from build123d import *
from build123d.topology import SkipClean

# Parameters (mm, degrees)
SKETCH1_R           = 15
SKETCH1_R_2         = 1.6
BOSS_EXTRUDE1_DEPTH = 7
BOSS_EXTRUDE2_DEPTH = 7.42
SKETCH3_R           = 9.5
BOSS_EXTRUDE3_DEPTH = 12.88
SKETCH5_R           = 1.6
CUT_EXTRUDE1_DEPTH  = 20
SKETCH6_R           = 2.75
CUT_EXTRUDE2_DEPTH  = 16
FILLET1_R           = 2
CHAMFER1_SIZE       = 0.4


with BuildPart() as part:
    # Sketch1 → Boss-Extrude1 (new body)
    with BuildSketch(Plane(origin=(0, 0, 0), x_dir=(1, 0, 0), z_dir=(0, 1, 0))):
        with Locations(Location((0, 0, 0), (0, 0, 270))):
            Circle(SKETCH1_R)
        with Locations(Location((0, 10, 0), (0, 0, 270))):
            Circle(SKETCH1_R_2, mode=Mode.SUBTRACT)
        with Locations(Location((0, -10, 0), (0, 0, 270))):
            Circle(SKETCH1_R_2, mode=Mode.SUBTRACT)
        with Locations(Location((10, 0, 0), (0, 0, 270))):
            Circle(SKETCH1_R_2, mode=Mode.SUBTRACT)
        with Locations(Location((-10, 0, 0), (0, 0, 270))):
            Circle(SKETCH1_R_2, mode=Mode.SUBTRACT)
    extrude(amount=BOSS_EXTRUDE1_DEPTH)

    # Sketch2 → Boss-Extrude2 (add)
    with BuildSketch(Plane(origin=(0, 7, 0), x_dir=(1, 0, 0), z_dir=(0, 1, 0))):
        Polygon((-6.505, 10.155), (6.505, 10.155), (10.155, 6.505), (10.155, -6.505), (6.505, -10.155), (-6.505, -10.155), (-10.155, -6.505), (-10.155, 6.505), align=None)
    extrude(amount=BOSS_EXTRUDE2_DEPTH)

    # Sketch3 → Boss-Extrude3 (add)
    with BuildSketch(Plane(origin=(0, 14.42, 0), x_dir=(1, 0, 0), z_dir=(0, 1, 0))):
        with Locations(Location((0, 0, 0), (0, 0, 90))):
            Circle(SKETCH3_R)
    extrude(amount=BOSS_EXTRUDE3_DEPTH)

    # Sketch4 → Cut-Revolve1 (revolve, cut)
    with BuildSketch(Plane.XY, mode=Mode.PRIVATE) as cut_revolve1_sk:
        Polygon((9, 25.05), (10, 25.05), (10, 26.05), (9.5, 26.05), (9, 25.761324865), align=None)
    revolve(cut_revolve1_sk.sketch.rotate(Axis((0, 27.3, 0), (0, -1, 0)), 270), axis=Axis((0, 27.3, 0), (0, -1, 0)), mode=Mode.SUBTRACT)

    # Sketch5 → Cut-Extrude1 (cut)
    with SkipClean():  # the faces are left unmerged after this step: merging them gives an invalid solid
        with BuildSketch(Plane.XZ):
            with Locations(Location((0, -10, 0), (0, 0, 185.559247246))):
                Circle(SKETCH5_R)
            with Locations(Location((10, 0, 0), (0, 0, 275.559247246))):
                Circle(SKETCH5_R)
            with Locations(Location((-10, 0, 0), (0, 0, 264.440752754))):
                Circle(SKETCH5_R)
            with Locations(Location((0, 10, 0), (0, 0, 202.624341254))):
                Circle(SKETCH5_R)
        extrude(amount=-CUT_EXTRUDE1_DEPTH, mode=Mode.SUBTRACT)

    # Sketch6 → Cut-Extrude2 (cut)
    with BuildSketch(Plane.XZ.offset(-20)):
        with Locations(Location((10, 0, 0), (0, 0, 90))):
            Circle(SKETCH6_R)
        with Locations(Location((0, 10, 0), (0, 0, 90))):
            Circle(SKETCH6_R)
        with Locations(Location((-10, 0, 0), (0, 0, 90))):
            Circle(SKETCH6_R)
        with Locations(Location((0, -10, 0), (0, 0, 90))):
            Circle(SKETCH6_R)
    extrude(amount=CUT_EXTRUDE2_DEPTH, mode=Mode.SUBTRACT)

    # Fillet1
    fillet1_edges = [part.edges().sort_by_distance(p)[0] for p in [
        (7.25, 20, 0),
        (0, 20, 7.25),
        (-7.25, 20, 0),
        (-1.609663202, 20, -7.770317427),
    ]]
    fillet(fillet1_edges, radius=FILLET1_R)

    # Chamfer1
    chamfer1_edges = [part.edges().sort_by_distance(p)[0] for p in [
        (0, 27.3, 9.5),
    ]]
    chamfer(chamfer1_edges, length=CHAMFER1_SIZE)


solid = part.part
Design review of the part built by this model. Coordinates are the model's own, in mm. A direction names the side the tool comes from. Round coordinates to 2 decimals unless told otherwise and drop trailing zeros. Order: outer loops, then holes, each group sorted by start corner. A loop starts at its lowest first (then second) coordinate and runs counter-clockwise, first axis right, second up.
1) For L1, parallel to Y at x = -5.75, z = -12; L2, parallel to X at y = 21.25, z = 0; L3, parallel to Y at x = 9.25, z = 5.5, list the stretches that pass through material, from the lowest coordinate up.
The answers:
L1: y = 0 to 7
L2: x = -9.5 to 9.5
L3: y = 0 to 14.42
2) Clearance check with flat-ended pins moving along their axes: pin 1 Ø8.5 at (x, z) = (7, 8) entering from +Y; pin 2 Ø3 at (x, y) = (4.5, 10) entering from -Z (3 decimals); pin 3 Ø8 at (x, y) = (2.5, 17) entering from +Z (3 decimals); pin 4 Ø3 at (y, z) = (9.5, -4) entering from -X (3 decimals). State where each tip first meets the part, or that it passes through.
The answers:
pin 1: stops at y = 27.3
pin 2: stops at z = -10.155
pin 3: stops at z = 10.155
pin 4: stops at x = -10.155
3) Consider section C-C (y = 16). State the section outline as (x, z) points, plus the area to 3 significant figures.
The answers:
outline: (-9.13, -2.61) arc R9.5 ccw to (-2.61, -9.13) arc R2.75 cw to (2.61, -9.13) arc R9.5 ccw to (9.13, -2.61) arc R2.75 cw to (9.13, 2.61) arc R9.5 ccw to (2.61, 9.13) arc R2.75 cw to (-2.61, 9.13) arc R9.5 ccw to (-9.13, 2.61) arc R2.75 cw to start
area: 250 mm2
4) Consider section D-D (y = 23.75). State the section outline as (x, z) points, plus the area to 3 significant figures.
The answers:
outline: circle Ø19 at (0, 0)
area: 284 mm2
5) Consider section A-A (z = 0). Count the separate pieces of the cut face and the enclosed holes in it, plus the area to 3 significant figures.
The answers:
separate pieces: 3
enclosed holes: 0
area: 479 mm2
6) Draft analysis for pull direction Y (two halves, no side actions). For faces 6 (the flat face through (10, 7, -7)), 7 (the flat face through (5, 11, -10.155)), 8 (the cylindrical face through (-0.83, 9.54, -7.38)), state which applies: released by +Y, released by -Y, zero draft, split by the parting line, or undercut.
The answers:
face 6: released by +Y
face 7: zero draft
face 8: undercut
7) Machinability: for faces 1 (the flat face through (-7, 14.42, 7)), 2 (the flat face through (-10.155, 11, -5)), 3 (the flat face through (-5, 11, 10.155)), 4 (the cylindrical face through (7.273, 9.542, -0.358)), 5 (the cylindrical face through (3.639, 19.661, -8.776)), which of the approach directions +Z, -Z, +X, -X, +Y, -Y give a long, thin tool a straight path to every point of the face, cutting with its end or side? Answer none if there is none.
The answers:
face 1: +Z, -X, +Y
face 2: +Z, -Z, -X, +Y
face 3: +Z, +X, -X, +Y
face 4: none
face 5: +Y
